Print and shaded views of the part. All mm, measured from the part's lowest x, y and z. A direction names the side the tool comes from. Round coordinates to 2 decimals unless told otherwise and drop trailing zeros. Write each loop counter-clockwise with the first axis right and the second up, starting at its lowest first coordinate (ties: lowest second). Pieces come first, ordered by that corner, then holes. Notation, with made-up numbers: (43.5, -33.75) -> (48.5, -33.75) arc R24 cw to (48.5, 1.25) -> close; hole circle Ø7 at (-39.75, -4.75). An arc over 180 degrees is marked (long way). Use CSV: the item, a comma, the result in double quotes. Start each with the question number.
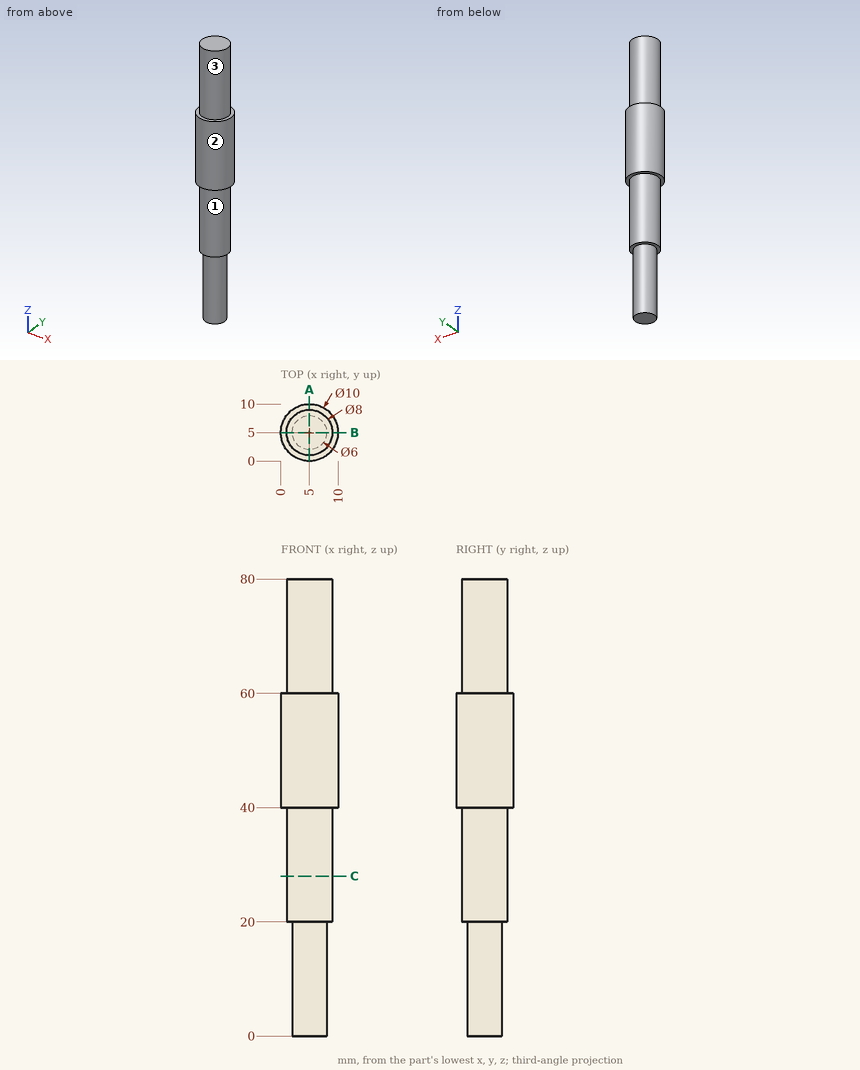
1. Band-saw the part on A-A (x = 5). List the corners of the cut face in (y, z).
2. Flat gauge pins, fed straight in: pin 1 (4 mm diameter, centred on y = 8, z = 18.5, fed in from +X); pin 2 (2 mm diameter, centred on x = 6.5, z = 15.5, fed in from +Y); pin 3 (4 mm diameter, centred on x = 4, z = 28, fed in from -Y). Where does each tip first touch, or does it go through?
3. Band-saw the part on C-C (z = 28). List the corners of the cut face in (x, y).
4. Drill centre lines: line 1 along Z through (x, y) = (7.5, 6.75); line 2 along Z through (x, y) = (9.75, 5.5); line 3 along Y through (x, z) = (7, 46). Where is each one in solid material? Low to high. Write a range as [from, to].
5. Which spindle directions (+Z, -Z, +X, -X, +Y, -Y) get a long thin tool onto all of the face, cutting with end or side? Do the marked faces 1, 2 and 3. Say none if no direction does.
Answers below:
1,outline,"(0, 40) -> (1, 40) -> (1, 20) -> (2, 20) -> (2, 0) -> (8, 0) -> (8, 20) -> (9, 20) -> (9, 40) -> (10, 40) -> (10, 60) -> (9, 60) -> (9, 80) -> (1, 80) -> (1, 60) -> (0, 60) -> close"
2,pin 1,"stops at x = 8.63"
2,pin 2,"stops at y = 7.96"
2,pin 3,"stops at y = 1"
3,outline,"circle Ø8 at (5, 5)"
4,line 1,"z = [20, 80]"
4,line 2,"z = [40, 60]"
4,line 3,"y = [0.42, 9.58]"
5,face 1,"-Z"
5,face 2,"+Z, -Z"
5,face 3,"+Z"
